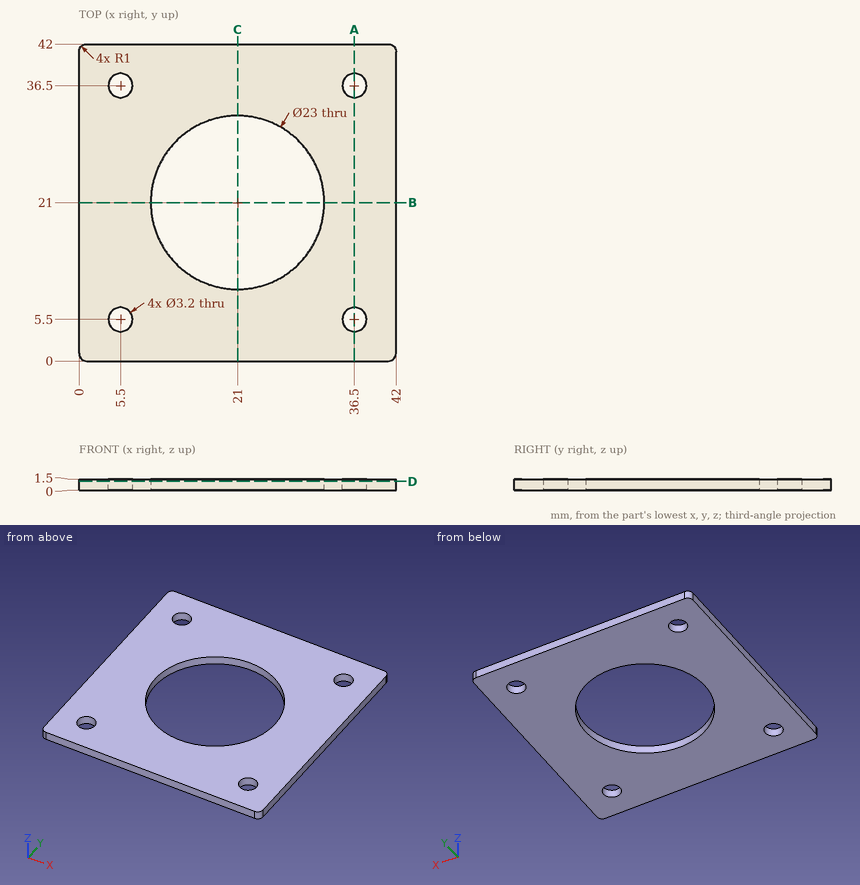
Answer from the drawing. Dimensions are ordinates in mm from the lowest x, y and z of the part. Coordinates: 2 decimals unless noted, no trailing zeros. Order: outer loops, then holes, each group sorted by start corner. A loop starts at its lowest first (then second) coordinate and runs counter-clockwise, first axis right, second up. Notation, with made-up numbers: (35, 46) - (82, 46) arc R16 cw to (82, 65) - close; hole circle Ø1 at (-25.75, 50.25). An arc over 180 degrees is marked (long way). Put each result on its own line as item: value. Start each with the question number.
1) Find section B-B (y = 21). Give the vertices of the cut face in (x, z), plus the area to 3 significant figures.
2) Find section A-A (x = 36.5). Give the vertices of the cut face in (y, z), plus the area to 3 significant figures.
3) Find the intervals of material crossed by line 1 (Y direction, x = 5.5, z = 0.85); line 2 (X direction, y = 21.5, z = 0.25); line 3 (Y direction, x = 37, z = 1.3), in increasing order. Write a range as from..to.
4) Find section D-D (z = 1.2). Give the vertices of the cut face in (x, y).
Results list:
1. outline: (0, 0) - (9.5, 0) - (9.5, 1.5) - (0, 1.5) - close; (32.5, 0) - (42, 0) - (42, 1.5) - (32.5, 1.5) - close
1. area: 28.5 mm^2
2. outline: (0, 0) - (3.9, 0) - (3.9, 1.5) - (0, 1.5) - close; (7.1, 0) - (34.9, 0) - (34.9, 1.5) - (7.1, 1.5) - close; (38.1, 0) - (42, 0) - (42, 1.5) - (38.1, 1.5) - close
2. area: 53.4 mm^2
3. line 1: y = 0..3.9, 7.1..34.9, 38.1..42
3. line 2: x = 0..9.51, 32.49..42
3. line 3: y = 0..3.98, 7.02..34.98, 38.02..42
4. outline: (0, 1) arc R1 ccw to (1, 0) - (41, 0) arc R1 ccw to (42, 1) - (42, 41) arc R1 ccw to (41, 42) - (1, 42) arc R1 ccw to (0, 41) - close; hole circle Ø3.2 at (5.5, 5.5); hole circle Ø3.2 at (5.5, 36.5); hole circle Ø23 at (21, 21); hole circle Ø3.2 at (36.5, 5.5); hole circle Ø3.2 at (36.5, 36.5)
